```python
from build123d import *

# Parameters (mm, degrees)
CROQUIS3_R               = 12.5
SALIENTE_EXTRUIR1_DEPTH  = 19
CROQUIS8_R               = 3.5
SALIENTE_EXTRUIR3_DEPTH  = 2.5
CROQUIS9_R               = 2
SALIENTE_EXTRUIR4_DEPTH  = 12.5
CROQUIS10_W              = 8
CROQUIS10_H              = 4
CORTAR_EXTRUIR5_DEPTH    = 5
CROQUIS11_R              = 1.5
CORTAR_EXTRUIR6_DEPTH    = 3
CROQUIS12_R              = 2
CORTAR_EXTRUIR7_DEPTH    = 3
CORTAR_EXTRUIR8_DEPTH    = 1.5
CORTAR_EXTRUIR9_DEPTH    = 1.5
REDONDEO1_R              = 0.25
CROQUIS16_W              = 1.05
CROQUIS16_H              = 0.3
SALIENTE_EXTRUIR5_DEPTH  = 4
CROQUIS17_R              = 4
SALIENTE_EXTRUIR6_DEPTH  = 0.75
SALIENTE_EXTRUIR7_START  = 0.75
CROQUIS18_R              = 3.5
SALIENTE_EXTRUIR7_DEPTH  = 0.75
CROQUIS19_R              = 11.6
SALIENTE_EXTRUIR8_DEPTH  = 2
CROQUIS20_R              = 1
SALIENTE_EXTRUIR9_DEPTH  = 4
CROQUIS21_R              = 7
SALIENTE_EXTRUIR10_DEPTH = 4
CROQUIS22_R              = 5
SALIENTE_EXTRUIR11_DEPTH = 0.5
CORTAR_EXTRUIR10_START   = -0.5
CROQUIS23_R              = 1
CORTAR_EXTRUIR10_DEPTH   = 0.5
SALIENTE_EXTRUIR12_DEPTH = 3
CORTAR_EXTRUIR11_DEPTH   = 3.5
CROQUIS26_R              = 0.75
SALIENTE_EXTRUIR13_DEPTH = 8
SALIENTE_EXTRUIR14_DEPTH = 6
CROQUIS28_W              = 5.4
CROQUIS28_H              = 2
SALIENTE_EXTRUIR15_DEPTH = 3


with BuildPart() as part:
    # Croquis1 → Revolución-Lámina1 (revolve)
    with BuildSketch(Plane.XY, mode=Mode.PRIVATE) as revoluci_n_l_mina1_sk:
        Polygon((0, 0), (0, 12.2), (30.8, 12.2), (30.8, 0), (20.8, 0), (20.8, 2.2), (10, 2.2), (10, 0), align=None)
    revolve(revoluci_n_l_mina1_sk.sketch.rotate(Axis((0, 0, 0), (1, 0, 0)), 90), axis=Axis((0, 0, 0), (1, 0, 0)))

    # Croquis3 → Saliente-Extruir1 (add)
    with BuildSketch(Plane.ZY):
        Circle(CROQUIS3_R)
    extrude(amount=SALIENTE_EXTRUIR1_DEPTH)

    # Croquis8 → Saliente-Extruir3 (add)
    with BuildSketch(Plane.ZY.offset(19)):
        Circle(CROQUIS8_R)
    extrude(amount=SALIENTE_EXTRUIR3_DEPTH)

    # Croquis9 → Saliente-Extruir4 (add)
    with BuildSketch(Plane.ZY.offset(19)):
        Circle(CROQUIS9_R)
    extrude(amount=SALIENTE_EXTRUIR4_DEPTH)

    # Croquis10 → Cortar-Extruir5 (cut)
    with BuildSketch(Plane.XY.offset(1)):
        with Locations((-27.5, 0)):
            Rectangle(CROQUIS10_W, CROQUIS10_H)
    extrude(amount=CORTAR_EXTRUIR5_DEPTH, mode=Mode.SUBTRACT)

    # Croquis11 → Cortar-Extruir6 (cut)
    with BuildSketch(Plane.ZY.offset(19)):
        with Locations((-8, 0)):
            Circle(CROQUIS11_R)
        with Locations((8, 0)):
            Circle(CROQUIS11_R)
    extrude(amount=-CORTAR_EXTRUIR6_DEPTH, mode=Mode.SUBTRACT)

    # Croquis12 → Cortar-Extruir7 (cut)
    with BuildSketch(Plane.ZY.offset(19)):
        with Locations((0, -8.5)):
            Circle(CROQUIS12_R)
        with Locations((0, 8.5)):
            Circle(CROQUIS12_R)
    extrude(amount=-CORTAR_EXTRUIR7_DEPTH, mode=Mode.SUBTRACT)

    # Croquis14 → Cortar-Extruir8 (cut)
    with BuildSketch(Plane.ZY.offset(16)):
        Polygon((-0.25, 8.25), (-0.25, 7.2), (0.25, 7.2), (0.25, 8.25), (1.3, 8.25), (1.3, 8.75), (0.25, 8.75), (0.25, 9.8), (-0.25, 9.8), (-0.25, 8.75), (-1.3, 8.75), (-1.3, 8.25), align=None)
    extrude(amount=-CORTAR_EXTRUIR8_DEPTH, mode=Mode.SUBTRACT)

    # Croquis15 → Cortar-Extruir9 (cut)
    with BuildSketch(Plane.ZY.offset(16)):
        Polygon((-0.25, -8.75), (-0.25, -9.8), (0.25, -9.8), (0.25, -8.75), (1.3, -8.75), (1.3, -8.25), (0.25, -8.25), (0.25, -7.2), (-0.25, -7.2), (-0.25, -8.25), (-1.3, -8.25), (-1.3, -8.75), align=None)
    extrude(amount=-CORTAR_EXTRUIR9_DEPTH, mode=Mode.SUBTRACT)

    # Redondeo1
    redondeo1_edges = [part.edges().sort_by_distance(p)[0] for p in [
        (-16, -8.5, -2),
        (-16, 8.5, -2),
    ]]
    fillet(redondeo1_edges, radius=REDONDEO1_R)

    # Croquis16 → Saliente-Extruir5 (add)
    with BuildSketch(Plane(origin=(30.8, 0, 0), x_dir=(0, 0, -1), z_dir=(1, 0, 0))):
        with Locations((-9.575, 0)):
            Rectangle(CROQUIS16_W, CROQUIS16_H)
        with Locations((8.525, 0)):
            Rectangle(CROQUIS16_W, CROQUIS16_H)
    extrude(amount=SALIENTE_EXTRUIR5_DEPTH)

    # Croquis17 → Saliente-Extruir6 (add)
    with BuildSketch(Plane(origin=(30.8, 0, 0), x_dir=(0, 0, -1), z_dir=(1, 0, 0))):
        Circle(CROQUIS17_R)
    extrude(amount=SALIENTE_EXTRUIR6_DEPTH)

    # Croquis18 → Saliente-Extruir7 (add)
    with BuildSketch(Plane(origin=(31.55, 0, 0), x_dir=(0, 0, -1), z_dir=(1, 0, 0)).offset(SALIENTE_EXTRUIR7_START)):
        with Locations(Location((0, 0, 0), (0, 0, 180))):
            Circle(CROQUIS18_R)
    extrude(amount=-SALIENTE_EXTRUIR7_DEPTH)

    # Croquis19 → Saliente-Extruir8 (add)
    with BuildSketch(Plane(origin=(32.3, 0, 0), x_dir=(0, 0, -1), z_dir=(1, 0, 0))):
        Circle(CROQUIS19_R)
    extrude(amount=SALIENTE_EXTRUIR8_DEPTH)

    # Croquis20 → Saliente-Extruir9 (add)
    with BuildSketch(Plane(origin=(34.3, 0, 0), x_dir=(0, 0, -1), z_dir=(1, 0, 0))):
        Circle(CROQUIS20_R)
    extrude(amount=SALIENTE_EXTRUIR9_DEPTH)

    # Croquis21 → Saliente-Extruir10 (add)
    with BuildSketch(Plane(origin=(38.3, 0, 0), x_dir=(0, 0, -1), z_dir=(1, 0, 0))):
        Circle(CROQUIS21_R)
    extrude(amount=SALIENTE_EXTRUIR10_DEPTH)

    # Croquis22 → Saliente-Extruir11 (add)
    with BuildSketch(Plane(origin=(42.3, 0, 0), x_dir=(0, 0, -1), z_dir=(1, 0, 0))):
        Circle(CROQUIS22_R)
    extrude(amount=SALIENTE_EXTRUIR11_DEPTH)

    # Croquis23 → Cortar-Extruir10 (cut)
    with BuildSketch(Plane(origin=(42.8, 0, 0), x_dir=(0, 0, -1), z_dir=(1, 0, 0)).offset(CORTAR_EXTRUIR10_START)):
        Circle(CROQUIS23_R)
    extrude(amount=CORTAR_EXTRUIR10_DEPTH, mode=Mode.SUBTRACT)

    # Croquis24 → Saliente-Extruir12 (add)
    with BuildSketch(Plane(origin=(34.3, 0, 0), x_dir=(0, 0, -1), z_dir=(1, 0, 0))):
        Polygon((0, 9.5), (6, 9.5), (6, 5.5), (-6, 5.5), (-6, 9.5), align=None)
    extrude(amount=SALIENTE_EXTRUIR12_DEPTH)

    # Croquis25 → Cortar-Extruir11 (cut)
    with BuildSketch(Plane(origin=(0, 9.5, 0), x_dir=(1, 0, 0), z_dir=(0, 1, 0))):
        Polygon((36.8, -5.5), (36.8, 5.5), (34.8, 5.5), (34.8, -5.5), (35.8, -5.5), align=None)
    extrude(amount=-CORTAR_EXTRUIR11_DEPTH, mode=Mode.SUBTRACT)

    # Croquis26 → Saliente-Extruir13 (add)
    with BuildSketch(Plane(origin=(0, 6, 0), x_dir=(1, 0, 0), z_dir=(0, 1, 0))):
        with Locations(Location((35.8, -4.4, 0), (0, 0, 270))):
            Circle(CROQUIS26_R)
        with Locations(Location((35.8, -2.8, 0), (0, 0, 270))):
            Circle(CROQUIS26_R)
        with Locations(Location((35.8, -0.8, 0), (0, 0, 270))):
            Circle(CROQUIS26_R)
        with Locations(Location((35.8, 0.8, 0), (0, 0, 270))):
            Circle(CROQUIS26_R)
        with Locations(Location((35.8, 2.8, 0), (0, 0, 270))):
            Circle(CROQUIS26_R)
        with Locations(Location((35.8, 4.4, 0), (0, 0, 270))):
            Circle(CROQUIS26_R)
    extrude(amount=SALIENTE_EXTRUIR13_DEPTH)

    # Croquis27 → Saliente-Extruir14 (add)
    with BuildSketch(Plane(origin=(34.3, 0, 0), x_dir=(0, 0, -1), z_dir=(1, 0, 0))):
        Polygon((0, -10.1), (3, -10.1), (3, -7.5), (-3, -7.5), (-3, -10.1), align=None)
    extrude(amount=SALIENTE_EXTRUIR14_DEPTH)

    # Croquis28 → Saliente-Extruir15 (add)
    with BuildSketch(Plane(origin=(40.3, 0, 0), x_dir=(0, 0, -1), z_dir=(1, 0, 0))):
        with Locations((0, -8.8)):
            Rectangle(CROQUIS28_W, CROQUIS28_H)
    extrude(amount=SALIENTE_EXTRUIR15_DEPTH)


solid = part.part
```
Work out the finished part from the listing and answer in its coordinate system (mm). A direction names the side the tool comes from. Coordinates: 2 decimals unless noted, no trailing zeros. Loops run counter-clockwise (first coordinate to the right, second up) from the corner with the lowest first, then second, coordinate; pieces in that order, holes last.
1) Consider probe 1 along Y at (x, z) = (-16.95, 0); probe 2 along X at (y, z) = (7, 5.25); probe 3 along X at (y, z) = (-8, 5.5). Determine where each line is inside the solid, lowest interval first.
Results:
probe 1: y = -12.5 to -10.5, -6.5 to 6.5, 10.5 to 12.5
probe 2: x = -19 to 30.8, 32.3 to 34.8, 36.8 to 37.3
probe 3: x = -19 to 30.8, 32.3 to 34.3
2) Flat-ended cylindrical pins translate along their axes: pin 1 (1 mm diameter, centred on y = 2.5, z = -8, fed in from -X); pin 2 (12 mm diameter, centred on x = 31.5, y = 7.5, fed in from +Z); pin 3 (5 mm diameter, centred on y = -7.5, z = -7, fed in from +X). Find the tip coordinate at first contact, or state that the pin passes through.
Results:
pin 1: stops at x = -19
pin 2: stops at z = 12.1
pin 3: stops at x = 34.3
3) Section A-A (z = -10.5) is taken. Give the vertices of the cut face in (x, y), plus the area to 3 significant figures.
Results:
outline: (-19, -6.78) - (0, -6.78) - (0, -6.21) - (30.8, -6.21) - (30.8, 6.21) - (0, 6.21) - (0, 6.78) - (-19, 6.78) - close; (32.3, -4.93) - (34.3, -4.93) - (34.3, 4.93) - (32.3, 4.93) - close
area: 660 mm2
4) Section C-C (x = -9) is taken. Give the vertices of the cut face in (y, z), plus the area to 3 significant figures.
Results:
outline: circle Ø25 at (0, 0)
area: 491 mm2
5) Section B-B (x = -20) is taken. Give the vertices of the cut face in (y, z).
Results:
outline: circle Ø7 at (0, 0)
6) For a pull along X with two mould halves and no side action, classify faces 1 (the cylindrical face through (15.32, -2.18, -0.29)), 2 (the flat face through (37, -9, -3)), 3 (the flat face through (-16, 8.1, 0.4)) as +X half, -X half, draft (parallel to the pull), parting line (faces both ways), or undercut.
Results:
face 1: undercut
face 2: draft
face 3: -X half
7) For faces 4 (the flat face through (37.3, 8, 0)), 5 (the cylindrical face through (35.135, 9.944, 4.746)), 6 (the flat face through (-21.5, -2, 2)), determine the directions among +Z, -Z, +X, -X, +Y, -Y from which every point of the face is accessible in a straight line to the end or side of a thin tool.
Results:
face 4: +Z, -Z, +Y
face 5: +Y
face 6: -X
